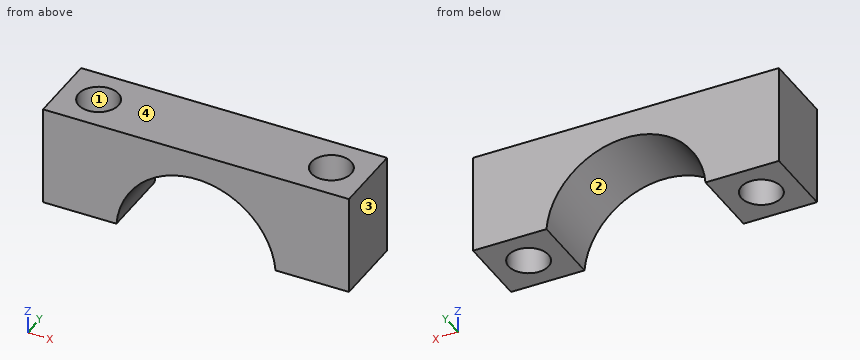
```python
from build123d import *

# Parameters (mm, degrees)
F2_DEPTH = 2.75
F4_D     = 3


with BuildPart() as f2:
    # F1 (on Front) → F2 (new body, symmetric)
    with BuildSketch(Plane.XZ):
        with BuildLine():
            ThreePointArc((-5.9791303716, 0.5), (0, 6), (5.9791303716, 0.5))
            Line((5.9791303716, 0.5), (11.5, 0.5))
            Line((11.5, 0.5), (11.5, 8))
            Line((11.5, 8), (-11.5, 8))
            Line((-11.5, 8), (-11.5, 0.5))
            Line((-11.5, 0.5), (-5.9791303716, 0.5))
        make_face()
    extrude(amount=F2_DEPTH, both=True)

    # F4 (through all)
    with Locations(Plane.XY.offset(8)):
        with Locations((-8.75, 0), (8.75, 0)):
            Hole(F4_D / 2)


solid = f2.part
```
Input: part model. Units: mm. Frame: model coordinates. Face numbers are marked on the shaded views. Round coordinates to 2 decimals unless told otherwise and drop trailing zeros. Order: outer loops, then holes, each group sorted by start corner. A loop starts at its lowest first (then second) coordinate and runs counter-clockwise, first axis right, second up. Notation, with made-up numbers: (52, -39.5) - (92, -39.5) arc R19 ccw to (92, -32.5) - close; hole circle Ø10 at (-6, 7.25). An arc over 180 degrees is marked (long way). One line per question, with ' | ' between items. Start each with the question number.
1) Ray query, probe 1 along Y at (x, z) = (8.75, 6); probe 2 along X at (y, z) = (0.95, 1.5); probe 3 along X at (y, z) = (0.35, 2). Return the intervals inside material, ascending.
2) Contact query for flat-ended pins moving along their axis: P1, Ø1.8, axis at x = 8.75, y = 0, coming from the -Z side; P2, Ø1.5, axis at x = 0.5, y = -1.5, coming from the -Z side. Output: stop coordinate, or through.
3) Cut plane C-C, the plane y = 0. Return the cut outline in (x, z), then the cut area to 3 significant figures.
4) Cut plane B-B, the plane z = 5.5. Return the cut outline in (x, y).
5) Cut plane A-A, the plane x = -8.75. Return the cut outline in (y, z), then the cut area to 4 significant figures.
6) Cut plane D-D, the plane y = -2.1. Return the cut outline in (x, z), then the cut area to 3 significant figures.
7) Pull-direction query (X, two-part tool) for the marked faces 1, 2, 3 and 4; classes: +X half, -X half, draft (parallel to the pull), parting line (faces both ways), or undercut.
Worked out:
1) probe 1: y = -2.75 to -1.5, 1.5 to 2.75 | probe 2: x = -11.5 to -9.91, -7.59 to -5.81, 5.81 to 7.59, 9.91 to 11.5 | probe 3: x = -11.5 to -10.21, -7.29 to -5.66, 5.66 to 7.29, 10.21 to 11.5
2) P1: passes through | P2: stops at z = 5.87
3) outline: (-11.5, 0.5) - (-10.25, 0.5) - (-10.25, 8) - (-11.5, 8) - close; (-7.25, 0.5) - (-5.98, 0.5) arc R6 cw to (5.98, 0.5) - (7.25, 0.5) - (7.25, 8) - (-7.25, 8) - close; (10.25, 0.5) - (11.5, 0.5) - (11.5, 8) - (10.25, 8) - close | area: 76.9 mm^2
4) outline: (-11.5, -2.75) - (-2.4, -2.75) - (-2.4, 2.75) - (-11.5, 2.75) - close; (2.4, -2.75) - (11.5, -2.75) - (11.5, 2.75) - (2.4, 2.75) - close; hole circle Ø3 at (-8.75, 0); hole circle Ø3 at (8.75, 0)
5) outline: (-2.75, 0.5) - (-1.5, 0.5) - (-1.5, 8) - (-2.75, 8) - close; (1.5, 0.5) - (2.75, 0.5) - (2.75, 8) - (1.5, 8) - close | area: 18.75 mm^2
6) outline: (-11.5, 0.5) - (-5.98, 0.5) arc R6 cw to (5.98, 0.5) - (11.5, 0.5) - (11.5, 8) - (-11.5, 8) - close | area: 122 mm^2
7) face 1: undercut | face 2: undercut | face 3: +X half | face 4: draft
